Design review of the part built by this model. Coordinates are the model's own, in mm. Face numbers are marked on the shaded views. Give positions to 0.01 mm unless a question says otherwise; leave off trailing zeros. Write each loop counter-clockwise with the first axis right and the second up, starting at its lowest first coordinate (ties: lowest second). Pieces come first, ordered by that corner, then holes. Notation, with made-up numbers: (-22, -30.75) -> (35, -30.75) arc R22 ccw to (35, -22.75) -> close; hole circle Ø9 at (-29.5, 73). An arc over 180 degrees is marked (long way). Answer as a JSON object with one key per item and string values.
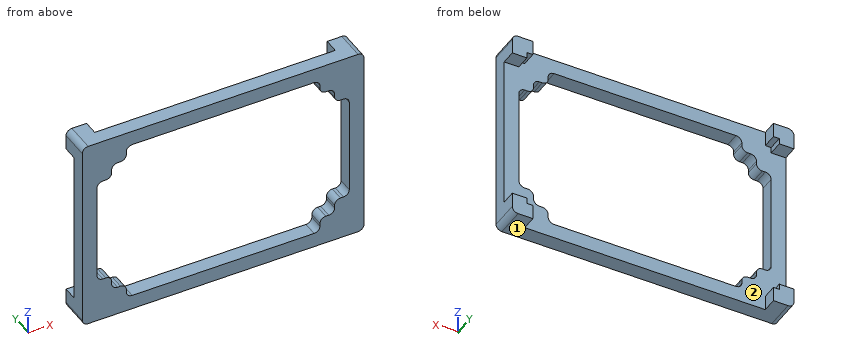
Autodesk Inventor part; units mm, degrees
ref_plane "YZ Plane" through (0, 0, 0) normal (1, 0, 0) x (0, 1, 0)
ref_plane "XZ Plane" through (0, 0, 0) normal (0, 1, 0) x (-1, 0, 0)
ref_plane "XY Plane" through (0, 0, 0) normal (0, 0, 1) x (1, 0, 0)
sketch "스케치2" plane through (0, 0, 0) normal (0, 1, 0) x (-1, 0, 0)
  line L0 (-43, 28.5) -> (43, 28.5)
  line L1 (43, 28.5) -> (43, -28.5)
  line L2 (43, -28.5) -> (-43, -28.5)
  line L3 (-43, -28.5) -> (-43, 28.5)
  line L4 (-43, 28.5) -> (43, -28.5) construction
  line L5 (43, 28.5) -> (-43, -28.5) construction
  line L6 (-48, -33.5) -> (48, -33.5)
  line L7 (48, -33.5) -> (48, 33.5)
  line L8 (48, 33.5) -> (-48, 33.5)
  line L9 (-48, 33.5) -> (-48, -33.5)
  point P0 (0, 0)
  dimension "d0" = 86
  dimension "d1" = 57
  dimension "d2" = 5
extrude "돌출1" add sketch "스케치2" against normal blind 5 contours L0 L1 L2 L3 | L9 L8 L7 L6
sketch "스케치5" plane through (0, 0, 0) normal (0, 1, 0) x (1, 0, 0)
  line L0 (-48, 33.5) -> (-48, -33.5)
  line L1 (-48, -33.5) -> (48, -33.5)
  line L2 (48, -33.5) -> (48, 33.5)
  line L3 (48, 33.5) -> (-48, 33.5)
  line L4 (-43, 28.5) -> (-43, -28.5)
  line L5 (-43, -28.5) -> (43, -28.5)
  line L6 (43, -28.5) -> (43, 28.5)
  line L7 (43, 28.5) -> (-43, 28.5)
  line L8 (-43, 28.5) -> (-33, 28.5)
  line L9 (-33, 28.5) -> (-33, 18.5)
  line L10 (-33, 18.5) -> (-43, 18.5)
  line L11 (-43, 18.5) -> (-43, 28.5)
  line L12 (-33, 18.5) -> (-38, 18.5)
  line L13 (-38, 18.5) -> (-38, 23.5)
  line L14 (-38, 23.5) -> (-33, 23.5)
  line L15 (-33, 23.5) -> (-33, 18.5)
  line L16 (-43, -28.5) -> (-33, -28.5)
  line L17 (-33, -28.5) -> (-33, -18.5)
  line L18 (-33, -18.5) -> (-43, -18.5)
  line L19 (-43, -18.5) -> (-43, -28.5)
  line L20 (-33, -18.5) -> (-38, -18.5)
  line L21 (-38, -18.5) -> (-38, -23.5)
  line L22 (-38, -23.5) -> (-33, -23.5)
  line L23 (-33, -23.5) -> (-33, -18.5)
  line L24 (43, -28.5) -> (33, -28.5)
  line L25 (33, -28.5) -> (33, -18.5)
  line L26 (33, -18.5) -> (43, -18.5)
  line L27 (43, -18.5) -> (43, -28.5)
  line L28 (33, -18.5) -> (38, -18.5)
  line L29 (38, -18.5) -> (38, -23.5)
  line L30 (38, -23.5) -> (33, -23.5)
  line L31 (33, -23.5) -> (33, -18.5)
  line L32 (43, 28.5) -> (33, 28.5)
  line L33 (33, 28.5) -> (33, 18.5)
  line L34 (33, 18.5) -> (43, 18.5)
  line L35 (43, 18.5) -> (43, 28.5)
  line L36 (33, 18.5) -> (38, 18.5)
  line L37 (38, 18.5) -> (38, 23.5)
  line L38 (38, 23.5) -> (33, 23.5)
  line L39 (33, 23.5) -> (33, 18.5)
  point P0 (0, 0)
  dimension "d10" = 5
  dimension "d11" = 10
  dimension "d12" = 10
  dimension "d13" = 5
  dimension "d14" = 5
  dimension "d15" = 10
  dimension "d16" = 10
  dimension "d17" = 5
  dimension "d18" = 5
  dimension "d19" = 10
  dimension "d20" = 10
  dimension "d21" = 5
  dimension "d22" = 5
  dimension "d23" = 10
  dimension "d24" = 10
  dimension "d25" = 5
  dimension "d26" = 5
extrude "돌출3" cut sketch "스케치5" against normal through all contours L10 L9 L7 L33 L34 L6 L26 L25 L5 L17 L18 L4 | L13 L14 L9 L10 | L18 L17 L22 L21 | L38 L37 L34 L33 | L25 L26 L29 L30
sketch "스케치3" plane through (0, 0, 0) normal (0, 1, 0) x (1, 0, 0)
  line L0 (-48, 33.5) -> (-48, -33.5)
  line L1 (-48, -33.5) -> (48, -33.5)
  line L2 (48, -33.5) -> (48, 33.5)
  line L3 (48, 33.5) -> (-48, 33.5)
  line L4 (-43, 28.5) -> (-43, -28.5)
  line L5 (-43, -28.5) -> (43, -28.5)
  line L6 (43, -28.5) -> (43, 28.5)
  line L7 (43, 28.5) -> (-43, 28.5)
  line L8 (-48, 26.5) -> (-43, 26.5)
  line L9 (-41, 33.5) -> (-41, 28.5)
  point P0 (0, 0)
  dimension "d5" = 5
  dimension "d6" = 7
  dimension "d7" = 7
extrude "돌출2" add sketch "스케치3" along normal blind 5 contours L3 L9 L7 L4 L8 L0
mirror "미러1" about plane through (0, 0, 0) normal (1, 0, 0) of "돌출2"
mirror "미러2" about plane through (0, 0, 0) normal (0, 0, 1) of "돌출2", "미러1"
fillet "모깎기1" radius 2 24 edges at (-33, -2.5, 28.5) (-33, -2.5, 23.5) (-38, -2.5, 23.5) (-38, -2.5, 18.5) (-43, -2.5, 18.5) (-48, 0, 33.5) (-48, 0, -33.5) (48, 0, -33.5) (48, 0, 33.5) (-43, -2.5, -18.5) (-38, -2.5, -18.5) (-38, -2.5, -23.5) (-33, -2.5, -23.5) (-33, -2.5, -28.5) (33, -2.5, -28.5) (33, -2.5, -23.5) (38, -2.5, -23.5) (38, -2.5, -18.5) (43, -2.5, -18.5) (43, -2.5, 18.5) (38, -2.5, 18.5) (38, -2.5, 23.5) (33, -2.5, 23.5) (33, -2.5, 28.5)
properties part number "Pi_Case"
(1) For line 1 along Z through (x, y) = (10, -0.75); line 2 along X through (y, z) = (1, 29); line 3 along X through (y, z) = (-3.75, 2.5), list the stretches that pass through material, from the lowest coordinate up.
Here are the results:
{"line 1": "z = -33.5 to -28.5, 28.5 to 33.5", "line 2": "x = -48 to -41, 41 to 48", "line 3": "x = -48 to -43, 43 to 48"}
(2) We need section A-A, the plane z = -11.5. State the section outline as (x, y) points, then the cut area to 3 significant figures.
Here are the results:
{"outline": "(-48, -5) -> (-43, -5) -> (-43, 0) -> (-48, 0) -> close; (43, -5) -> (48, -5) -> (48, 0) -> (43, 0) -> close", "area": "50.0 mm²"}
(3) We need section C-C, the plane y = 1.25. State the section outline as (x, z) points, then the cut area to 3 significant figures.
Here are the results:
{"outline": "(-48, -31.5) arc R2 ccw to (-46, -33.5) -> (-41, -33.5) -> (-41, -28.5) -> (-43, -28.5) -> (-43, -26.5) -> (-48, -26.5) -> close; (-48, 26.5) -> (-43, 26.5) -> (-43, 28.5) -> (-41, 28.5) -> (-41, 33.5) -> (-46, 33.5) arc R2 ccw to (-48, 31.5) -> close; (41, -33.5) -> (46, -33.5) arc R2 ccw to (48, -31.5) -> (48, -26.5) -> (43, -26.5) -> (43, -28.5) -> (41, -28.5) -> close; (41, 28.5) -> (43, 28.5) -> (43, 26.5) -> (48, 26.5) -> (48, 31.5) arc R2 ccw to (46, 33.5) -> (41, 33.5) -> close", "area": "177 mm²"}
(4) The part is to be moulded in two halves that separate along X. For the marked faces 1 and 2, say which applies: +X half, -X half, draft (parallel to the pull), parting line (faces both ways), or undercut.
Here are the results:
{"face 1": "draft", "face 2": "undercut"}
(5) We need section D-D, the plane z = 27.5. State the section outline as (x, y) points.
Here are the results:
{"outline": "(-48, -5) -> (-32.73, -5) -> (-32.73, 0) -> (-43, 0) -> (-43, 5) -> (-48, 5) -> close; (32.73, -5) -> (48, -5) -> (48, 5) -> (43, 5) -> (43, 0) -> (32.73, 0) -> close"}
(6) We need section B-B, the plane x = -28. State the section outline as (y, z) points, then the cut area to 3 significant figures.
Here are the results:
{"outline": "(-5, -33.5) -> (0, -33.5) -> (0, -28.5) -> (-5, -28.5) -> close; (-5, 28.5) -> (0, 28.5) -> (0, 33.5) -> (-5, 33.5) -> close", "area": "50.0 mm²"}
